Can you work these out from the model? Positions are in its coordinate system, mm. A direction names the side the tool comes from. Round coordinates to 2 decimals unless told otherwise and drop trailing zeros. Loops run counter-clockwise (first coordinate to the right, second up) from the corner with the lowest first, then second, coordinate; pieces in that order, holes last. Notation, with made-up numbers: (41.5, 42.25) - (100.5, 42.25) arc R17 cw to (100.5, 72.25) - close; hole circle Ø5 at (58, 17). An arc over 180 degrees is marked (long way). Answer as CSV lines item,"result".
```python
from build123d import *

# Parameters (mm, degrees)
SKETCH_4_W          = 23.5
SKETCH_4_H          = 56
EXTRUDE_1_DEPTH     = 3
SKETCH_5_R          = 0.75
CUT_EXTRUDE_1_DEPTH = 37.67764987
SKETCH_5_3_R        = 1.5
CUT_EXTRUDE_4_DEPTH = 1.2
CUT_EXTRUDE_START   = -22.3
SKETCH_5_4_R        = 1.5
CUT_EXTRUDE_5_DEPTH = 1.2
SKETCH_6_R          = 1.5
SKETCH_6_R_2        = 1
CUT_EXTRUDE_2_DEPTH = 1
SKETCH_6_2_R        = 1
CUT_EXTRUDE_3_DEPTH = 31.513316765
SKETCH_7_W          = 44
SKETCH_7_H          = 3
CUT_EXTRUDE_8_DEPTH = 0.5
CUT_EXTRUDE_START_2 = -23.5
SKETCH_7_2_W        = 44
SKETCH_7_2_H        = 3
CUT_EXTRUDE_9_DEPTH = 0.5


with BuildPart() as part:
    # 草图4 → 凸台-拉伸1 (new body)
    with BuildSketch(Plane(origin=(0, 0, 0), x_dir=(1, 0, 0), z_dir=(0, 1, 0))):
        Rectangle(SKETCH_4_W, SKETCH_4_H)
    extrude(amount=EXTRUDE_1_DEPTH)

    # 草图5 → 切除-拉伸1 (cut, through all)
    with BuildSketch(Plane(origin=(11.75, 0, 0), x_dir=(0, 0, -1), z_dir=(1, 0, 0))):
        with Locations((-25, 3)):
            Circle(SKETCH_5_R)
        with Locations((25, 3)):
            Circle(SKETCH_5_R)
    extrude(amount=-CUT_EXTRUDE_1_DEPTH, mode=Mode.SUBTRACT)

    # 草图5<3> → 切除-拉伸4 (cut)
    with BuildSketch(Plane(origin=(11.75, 0, 0), x_dir=(0, 0, -1), z_dir=(1, 0, 0))):
        with Locations((-25, 3)):
            Circle(SKETCH_5_3_R)
        with Locations((25, 3)):
            Circle(SKETCH_5_3_R)
    extrude(amount=-CUT_EXTRUDE_4_DEPTH, mode=Mode.SUBTRACT)

    # 草图5<4> → 切除-拉伸5 (cut)
    with BuildSketch(Plane(origin=(11.75, 0, 0), x_dir=(0, 0, -1), z_dir=(1, 0, 0)).offset(CUT_EXTRUDE_START)):
        with Locations((-25, 3)):
            Circle(SKETCH_5_4_R)
        with Locations((25, 3)):
            Circle(SKETCH_5_4_R)
    extrude(amount=-CUT_EXTRUDE_5_DEPTH, mode=Mode.SUBTRACT)

    # 草图6 → 切除-拉伸2 (cut)
    # profile 1 of 4: a face of its own
    with BuildSketch(Plane.XZ):
        with Locations(Location((-9.25, -20, 0), (0, 0, 270))):
            Circle(SKETCH_6_R)
        with Locations(Location((-9.25, -20, 0), (0, 0, 270))):
            Circle(SKETCH_6_R_2, mode=Mode.SUBTRACT)
    # profile 2 of 4: a face of its own
    with BuildSketch(Plane.XZ):
        with Locations(Location((9.25, -20, 0), (0, 0, 270))):
            Circle(SKETCH_6_R)
        with Locations(Location((9.25, -20, 0), (0, 0, 270))):
            Circle(SKETCH_6_R_2, mode=Mode.SUBTRACT)
    # profile 3 of 4: a face of its own
    with BuildSketch(Plane.XZ):
        with Locations(Location((-9.25, 20, 0), (0, 0, 270))):
            Circle(SKETCH_6_R)
        with Locations(Location((-9.25, 20, 0), (0, 0, 270))):
            Circle(SKETCH_6_R_2, mode=Mode.SUBTRACT)
    # profile 4 of 4: a face of its own
    with BuildSketch(Plane.XZ):
        with Locations(Location((9.25, 20, 0), (0, 0, 270))):
            Circle(SKETCH_6_R)
        with Locations(Location((9.25, 20, 0), (0, 0, 270))):
            Circle(SKETCH_6_R_2, mode=Mode.SUBTRACT)
    extrude(amount=-CUT_EXTRUDE_2_DEPTH, mode=Mode.SUBTRACT)

    # 草图6<2> → 切除-拉伸3 (cut, through all)
    with BuildSketch(Plane.XZ):
        with Locations(Location((-9.25, -20, 0), (0, 0, 270))):
            Circle(SKETCH_6_2_R)
        with Locations(Location((9.25, -20, 0), (0, 0, 270))):
            Circle(SKETCH_6_2_R)
        with Locations(Location((-9.25, 20, 0), (0, 0, 270))):
            Circle(SKETCH_6_2_R)
        with Locations(Location((9.25, 20, 0), (0, 0, 270))):
            Circle(SKETCH_6_2_R)
    extrude(amount=-CUT_EXTRUDE_3_DEPTH, mode=Mode.SUBTRACT)

    # 草图7 → 切除-拉伸8 (cut)
    with BuildSketch(Plane.ZY.offset(11.75)):
        with Locations((0, 1.5)):
            Rectangle(SKETCH_7_W, SKETCH_7_H)
    extrude(amount=-CUT_EXTRUDE_8_DEPTH, mode=Mode.SUBTRACT)

    # 草图7<2> → 切除-拉伸9 (cut)
    with BuildSketch(Plane.ZY.offset(11.75).offset(CUT_EXTRUDE_START_2)):
        with Locations((0, 1.5)):
            Rectangle(SKETCH_7_2_W, SKETCH_7_2_H)
    extrude(amount=CUT_EXTRUDE_9_DEPTH, mode=Mode.SUBTRACT)


solid = part.part
```
Q1. Imagine slicing it at A-A (z = 20). Write out the boundary of the cut face in (x, y), then the cut area to 3 significant figures.
Checks:
outline,"(-11.25, 0) - (-10.75, 0) - (-10.75, 1) - (-10.25, 1) - (-10.25, 3) - (-11.25, 3) - close; (-8.25, 1) - (-7.75, 1) - (-7.75, 0) - (7.75, 0) - (7.75, 1) - (8.25, 1) - (8.25, 3) - (-8.25, 3) - close; (10.25, 1) - (10.75, 1) - (10.75, 0) - (11.25, 0) - (11.25, 3) - (10.25, 3) - close"
area,"53.5 mm²"
Q2. Imagine slicing it at C-C (y = 0.5). Write out the boundary of the cut face in (x, z), then the cut area to 3 significant figures.
Checks:
outline,"(-11.75, -28) - (11.75, -28) - (11.75, -22) - (11.25, -22) - (11.25, 22) - (11.75, 22) - (11.75, 28) - (-11.75, 28) - (-11.75, 22) - (-11.25, 22) - (-11.25, -22) - (-11.75, -22) - close; hole circle Ø3 at (-9.25, -20); hole circle Ø3 at (-9.25, 20); hole circle Ø3 at (9.25, -20); hole circle Ø3 at (9.25, 20)"
area,"1,240 mm²"
Q3. We'd pull the mould along Z, two halves only. Please class faces 1 (the flat face through (0, 1, 28)), 2 (the cylindrical face through (9.3, 0.5, -18.5)), 3 (the flat face through (0, 3, 0)): pulls with the +Z half, pulls with the -Z half, needs draft (parallel to the pull), parting line crosses it, or undercut.
Checks:
face 1,"pulls with the +Z half"
face 2,"undercut"
face 3,"needs draft"
Q4. If I drill on line 1 along X through (y, z) = (0.3, -20); line 2 along X through (y, z) = (2.4, -20); line 3 along Z through (x, y) = (-9.75, 1.85), over which ranges is the centre line in solid material (lowest first)? Write a range as [from, to].
Checks:
line 1,"[-11.25, -10.75], [-7.75, 7.75], [10.75, 11.25]"
line 2,"[-11.25, -10.25], [-8.25, 8.25], [10.25, 11.25]"
line 3,"[-28, -20.87], [-19.13, 19.13], [20.87, 28]"
Q5. I'm going to push flat-ended pins straight in: pin 1 Ø1.5 at (x, z) = (-9, 20.5) entering from -Y; pin 2 Ø1 at (y, z) = (2, 8) entering from -X; pin 3 Ø1.5 at (y, z) = (2.5, 10) entering from +X; pin 4 Ø1.6 at (x, z) = (-9.25, 20) entering from -Y. Where does each tip first touch, or does it pass through?
Checks:
pin 1,"y = 1"
pin 2,"x = -11.25"
pin 3,"x = 11.25"
pin 4,"through"
Q6. Imagine slicing it at D-D (z = -25). Write out the boundary of the cut face in (x, y), then the cut area to 3 significant figures.
Checks:
outline,"(-11.75, 0) - (11.75, 0) - (11.75, 1.5) - (10.55, 1.5) - (10.55, 2.25) - (-10.55, 2.25) - (-10.55, 1.5) - (-11.75, 1.5) - close"
area,"51.1 mm²"
Q7. Imagine slicing it at B-B (x = -9.25). Write out the boundary of the cut face in (y, z), then the cut area to 3 significant figures.
Checks:
outline,"(0, -28) - (3, -28) - (3, -25.75) arc R0.75 cw to (3, -24.25) - (3, -21) - (1, -21) - (1, -21.5) - (0, -21.5) - close; (0, -18.5) - (1, -18.5) - (1, -19) - (3, -19) - (3, 19) - (1, 19) - (1, 18.5) - (0, 18.5) - close; (0, 21.5) - (1, 21.5) - (1, 21) - (3, 21) - (3, 24.25) arc R0.75 cw to (3, 25.75) - (3, 28) - (0, 28) - close"
area,"152 mm²"
Q8. On a 3-axis mill with a long thin cutter (end or side, diameter ignored), from which of +Z, -Z, +X, -X, +Y, -Y can I reach the whole of each face in a straight line? I mean faces 4 (the flat face through (-10, 1, 19)), 5 (the flat face through (-11.25, 2, 0)), 6 (the flat face through (-10.55, 2, 25)). Say none if no direction works.
Checks:
face 4,"-Y"
face 5,"-X, +Y, -Y"
face 6,"-X, +Y"
